from build123d import *

# Parameters (mm, degrees)
SKETCH1_R           = 22.2
BOSS_EXTRUDE1_DEPTH = 1
BOSS_EXTRUDE2_START = 1
SKETCH2_R           = 11.25
BOSS_EXTRUDE2_DEPTH = 8.5
BOSS_EXTRUDE3_START = 9.5
SKETCH3_R           = 5
BOSS_EXTRUDE3_DEPTH = 9.5
CUT_EXTRUDE1_START  = 19
SKETCH4_W           = 11.621745696
SKETCH4_H           = 1
CUT_EXTRUDE1_DEPTH  = 9.5
BOSS_EXTRUDE4_START = 1
SKETCH5_R           = 3.5
BOSS_EXTRUDE4_DEPTH = 3
SKETCH6_R           = 6
CUT_EXTRUDE2_DEPTH  = 3.5
SKETCH9_R           = 8.35
BOSS_EXTRUDE5_DEPTH = 5
CUT_EXTRUDE7_START  = -2
SKETCH10_R          = 11.25
SKETCH10_R_2        = 8.35
CUT_EXTRUDE7_DEPTH  = 3.5
SKETCH11_R          = 0.75
CUT_EXTRUDE8_DEPTH  = 3


with BuildPart() as part:
    # Sketch1 → Boss-Extrude1 (new body)
    with BuildSketch(Plane.XY):
        Circle(SKETCH1_R)
    extrude(amount=BOSS_EXTRUDE1_DEPTH)

    # Sketch2 → Boss-Extrude2 (add)
    with BuildSketch(Plane.XY.offset(BOSS_EXTRUDE2_START)):
        Circle(SKETCH2_R)
    extrude(amount=BOSS_EXTRUDE2_DEPTH)

    # Sketch3 → Boss-Extrude3 (add)
    with BuildSketch(Plane.XY.offset(BOSS_EXTRUDE3_START)):
        Circle(SKETCH3_R)
    extrude(amount=BOSS_EXTRUDE3_DEPTH)

    # Sketch4 → Cut-Extrude1 (cut)
    with BuildSketch(Plane.XY.offset(CUT_EXTRUDE1_START)):
        Rectangle(SKETCH4_W, SKETCH4_H)
    extrude(amount=-CUT_EXTRUDE1_DEPTH, mode=Mode.SUBTRACT)

    # Sketch5 → Boss-Extrude4 (add)
    with BuildSketch(Plane.XY.offset(BOSS_EXTRUDE4_START)):
        with Locations((0, 16.6)):
            Circle(SKETCH5_R)
    extrude(amount=BOSS_EXTRUDE4_DEPTH)

    # Sketch6 → Cut-Extrude2 (cut)
    with BuildSketch(Plane(origin=(0, 0, 0), x_dir=(-1, 0, 0), z_dir=(0, 0, -1))):
        Circle(SKETCH6_R)
    extrude(amount=-CUT_EXTRUDE2_DEPTH, mode=Mode.SUBTRACT)

    # Sketch9 → Boss-Extrude5 (add)
    with BuildSketch(Plane.XY.offset(19)):
        Circle(SKETCH9_R)
    extrude(amount=-BOSS_EXTRUDE5_DEPTH)

    # Sketch10 → Cut-Extrude7 (cut)
    with BuildSketch(Plane.XY.offset(9.5).offset(CUT_EXTRUDE7_START)):
        Circle(SKETCH10_R)
        Circle(SKETCH10_R_2, mode=Mode.SUBTRACT)
    extrude(amount=-CUT_EXTRUDE7_DEPTH, mode=Mode.SUBTRACT)

    # Sketch11 → Cut-Extrude8 (cut)
    with BuildSketch(Plane.XY.offset(9.5)):
        with Locations((9.495112761, -0.304686158)):
            Circle(SKETCH11_R)
    extrude(amount=-CUT_EXTRUDE8_DEPTH, mode=Mode.SUBTRACT)


solid = part.part
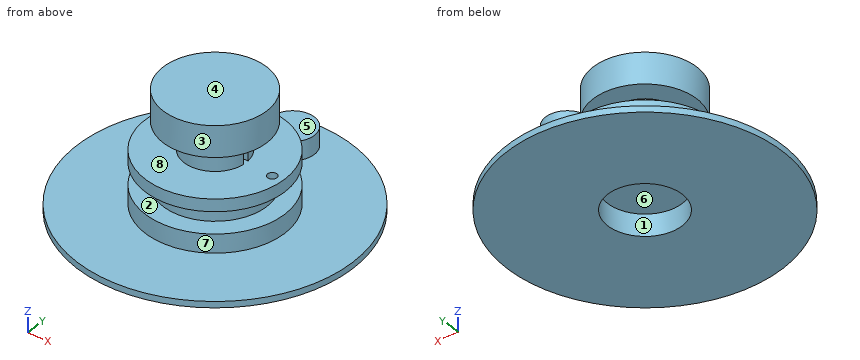
CAD build for the part. Positions are in the model's coordinates, mm. Face numbers are marked on the shaded views. A direction names the side the tool comes from. Give positions to 0.01 mm unless a question says otherwise; leave off trailing zeros. Write each loop counter-clockwise with the first axis right and the second up, starting at its lowest first coordinate (ties: lowest second). Pieces come first, ordered by that corner, then holes. Notation, with made-up numbers: (69, 51) -> (115, 51) arc R13 ccw to (115, 69) -> close; hole circle Ø9 at (74, 19.25). An arc over 180 degrees is marked (long way). Return JSON: item names as keys, results as strings.
Item 1: Band-saw the part on C-C (z = 17.5). List the corners of the cut face in (x, y), then the cut area to 3 significant figures.
Answer below:
{"outline": "circle Ø16.7 at (0, 0)", "area": "219 mm2"}
Item 2: Two-plate mould, pull along Y, no slides. Class the marked faces 1, 2 and 3: +Y half, -Y half, draft (parallel to the pull), parting line (faces both ways), or undercut.
Answer below:
{"face 1": "undercut", "face 2": "draft", "face 3": "parting line"}
Item 3: Band-saw the part on B-B (y = -9). List the corners of the cut face in (x, z).
Answer below:
{"outline": "(-20.29, 0) -> (20.29, 0) -> (20.29, 1) -> (6.75, 1) -> (6.75, 4) -> (-6.75, 4) -> (-6.75, 1) -> (-20.29, 1) -> close; (-6.75, 7.5) -> (6.75, 7.5) -> (6.75, 9.5) -> (-6.75, 9.5) -> close"}
Item 4: Tool access for the marked faces 4, 5, 6, 7 and 8: list every direction of +Z, -Z, +X, -X, +Y, -Y with a clear straight run to the whole face (end or side of a thin tool).
Answer below:
{"face 4": "+Z, +X, -X, +Y, -Y", "face 5": "+Z, +X, -X, +Y", "face 6": "-Z", "face 7": "+Z", "face 8": "none"}
Item 5: Band-saw the part on A-A (x = 7.5). List the corners of the cut face in (y, z).
Answer below:
{"outline": "(-20.89, 0) -> (20.89, 0) -> (20.89, 1) -> (8.39, 1) -> (8.39, 4) -> (3.67, 4) -> (3.67, 7.5) -> (8.39, 7.5) -> (8.39, 9.5) -> (-8.39, 9.5) -> (-8.39, 7.5) -> (-3.67, 7.5) -> (-3.67, 4) -> (-8.39, 4) -> (-8.39, 1) -> (-20.89, 1) -> close; (-3.67, 14) -> (3.67, 14) -> (3.67, 19) -> (-3.67, 19) -> close"}
Item 6: Drill centre lines: probe 1 along Y at (x, z) = (0, 1.35); probe 2 along Z at (x, y) = (0.5, 8); probe 3 along Y at (x, z) = (0, 14.5). Where is each one in solid material? Low to high.
Answer below:
{"probe 1": "y = -11.25 to -6, 6 to 11.25, 13.1 to 20.1", "probe 2": "z = 0 to 9.5, 14 to 19", "probe 3": "y = -8.35 to 8.35"}
Item 7: Band-saw the part on D-D (y = 4). List the corners of the cut face in (x, z).
Answer below:
{"outline": "(-21.84, 0) -> (-4.47, 0) -> (-4.47, 3.5) -> (4.47, 3.5) -> (4.47, 0) -> (21.84, 0) -> (21.84, 1) -> (10.51, 1) -> (10.51, 4) -> (7.33, 4) -> (7.33, 7.5) -> (10.51, 7.5) -> (10.51, 9.5) -> (3, 9.5) -> (3, 14) -> (7.33, 14) -> (7.33, 19) -> (-7.33, 19) -> (-7.33, 14) -> (-3, 14) -> (-3, 9.5) -> (-10.51, 9.5) -> (-10.51, 7.5) -> (-7.33, 7.5) -> (-7.33, 4) -> (-10.51, 4) -> (-10.51, 1) -> (-21.84, 1) -> close"}
Item 8: Drop flat-ended pins along their axis: pin 1 (3 mm diameter, centred on x = -3.5, z = 13, fed in from +Y); pin 2 (3.5 mm diameter, centred on x = 1.5, y = 16.5, fed in from +Z); pin 3 (5 mm diameter, centred on x = -0.5, z = 12.5, fed in from -Y). Give the stop position or say it passes through.
Answer below:
{"pin 1": "stops at y = 8", "pin 2": "stops at z = 4", "pin 3": "stops at y = -8.35"}
